```python
from build123d import *

# Parameters (mm, degrees)
F2_DEPTH = 16.5
F3_DEPTH = 21


with BuildPart() as f2:
    # F1 (on face) → F2 (new body)
    with BuildSketch(Plane.XY):
        with BuildLine():
            Line((-40, -47), (40, -47))
            ThreePointArc((40, -47), (71.819805, -33.819805), (85, -2))
            Line((85, -2), (85, 2))
            ThreePointArc((85, 2), (71.819805, 33.819805), (40, 47))
            Line((40, 47), (-40, 47))
            ThreePointArc((-40, 47), (-71.819805, 33.819805), (-85, 2))
            Line((-85, 2), (-85, -2))
            ThreePointArc((-85, -2), (-71.819805, -33.819805), (-40, -47))
        make_face()
    extrude(amount=F2_DEPTH)

    # F0 (on Top) → F3 (intersect)
    with BuildSketch(Plane.XY):
        with BuildLine():
            Line((-44.5, -51.5), (44.5, -51.5))
            ThreePointArc((44.5, -51.5), (76.319805, -38.319805), (89.5, -6.5))
            Line((89.5, -6.5), (89.5, 6.5))
            ThreePointArc((89.5, 6.5), (76.319805, 38.319805), (44.5, 51.5))
            Line((44.5, 51.5), (-44.5, 51.5))
            ThreePointArc((-44.5, 51.5), (-76.319805, 38.319805), (-89.5, 6.5))
            Line((-89.5, 6.5), (-89.5, -6.5))
            ThreePointArc((-89.5, -6.5), (-76.319805, -38.319805), (-44.5, -51.5))
        make_face()
    extrude(amount=F3_DEPTH, mode=Mode.INTERSECT)


solid = f2.part
```
The model under review builds one solid part; all positions refer to its coordinate system, in mm. Round coordinates to 2 decimals unless told otherwise and drop trailing zeros. Order: outer loops, then holes, each group sorted by start corner. A loop starts at its lowest first (then second) coordinate and runs counter-clockwise, first axis right, second up.
(1) Wall thickness on L1, parallel to X at y = -17, z = 13.25; L2, parallel to Y at x = -66.5, z = 13.75; L3, parallel to X at y = 20, z = 6.25: over which ranges is each line inside the solid? List them lowest first.
Working result:
L1: x = -82.43 to 82.43
L2: y = -38.37 to 38.37
L3: x = -81.24 to 81.24
(2) Take a section at B-B, the plane x = 72. State the section outline as (y, z) points, plus the area to 3 significant figures.
Working result:
outline: (-33.64, 0) - (33.64, 0) - (33.64, 16.5) - (-33.64, 16.5) - close
area: 1,110 mm2
(3) Take a section at C-C, the plane y = -25.5. State the section outline as (x, z) points.
Working result:
outline: (-78.38, 0) - (78.38, 0) - (78.38, 16.5) - (-78.38, 16.5) - close
(4) For P1, Ø3, axis at x = 54, z = 12.5, coming from the -Y side; P2, Ø4, axis at x = 33.5, y = -5.5, coming from the -Z side; P3, Ø1, axis at y = -27.5, z = 4.5, coming from the +X side, all flat-tipped, find the tip position at first contact; note any pin that passes through.
Working result:
P1: stops at y = -45.23
P2: stops at z = 0
P3: stops at x = 77.42
(5) Take a section at A-A, the plane z = 6.25. State the section outline as (x, y) points, plus the area to 3 significant figures.
Working result:
outline: (-85, -2) arc R45 ccw to (-40, -47) - (40, -47) arc R45 ccw to (85, -2) - (85, 2) arc R45 ccw to (40, 47) - (-40, 47) arc R45 ccw to (-85, 2) - close
area: 14,200 mm2
(6) Mouldability with a two-part tool opening along X and no side actions: class faces 1 (the face through (72.168, 33.468, 8.134)), 2 (the face through (-1, -47, 8)), 3 (the face through (-72.168, -33.468, 8.134)) as released by +X, released by -X, zero draft, split by the parting line, or undercut.
Working result:
face 1: released by +X
face 2: zero draft
face 3: released by -X
